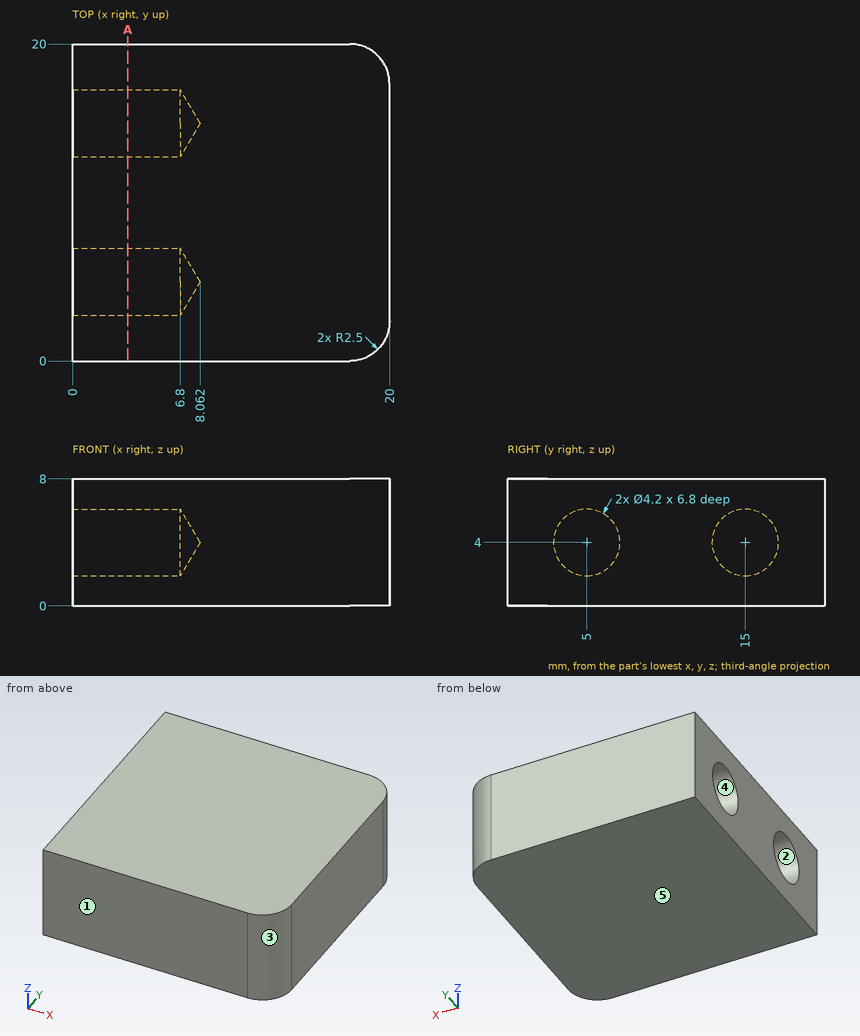
Verification items for this drawing (mm, ordinates from the low corner). A direction names the side the tool comes from. Coordinates: 2 decimals unless noted, no trailing zeros. Order: outer loops, then holes, each group sorted by start corner. A loop starts at its lowest first (then second) coordinate and runs counter-clockwise, first axis right, second up. Notation, with made-up numbers: (-5.75, 66.25) -> (35.25, 66.25) arc R13 cw to (35.25, 91.25) -> close; hole circle Ø6 at (-0.75, -30). An arc over 180 degrees is marked (long way). Answer as CSV lines item,"result". Start each with the question number.
1) Material ranges on L1, parallel to Y at x = 2, z = 4; L2, parallel to Z at x = 4, y = 15; L3, parallel to Z at x = 7.5, y = 14.5, recorded low to high. Write a range as [from, to].
2) Release check for a two-part mould opening along Y. For the marked faces 3, 4 and 5 record: released by +Y, released by -Y, zero draft, split by the parting line, or undercut.
3) Set-up check for the marked faces 1 and 2: record each of +Z, -Z, +X, -X, +Y, -Y from which the full face is reachable in a straight line by a thin tool's end or side.
4) Cross-section at A-A, the plane x = 3.5. Record the boundary of the cut face in (y, z).
5) Gauge pin test, flat ends, axial feed: pin 1 Ø1 at (y, z) = (18, 2) entering from -X; pin 2 Ø3.5 at (y, z) = (15, 4) entering from -X. Record the tip position at first contact, or that the pin passes through.
Conclusion:
1,L1,"y = [0, 2.9], [7.1, 12.9], [17.1, 20]"
1,L2,"z = [0, 1.9], [6.1, 8]"
1,L3,"z = [0, 3.21], [4.79, 8]"
2,face 3,"released by -Y"
2,face 4,"undercut"
2,face 5,"zero draft"
3,face 1,"+Z, -Z, +X, -X, -Y"
3,face 2,"-X"
4,outline,"(0, 0) -> (20, 0) -> (20, 8) -> (0, 8) -> close; hole circle Ø4.2 at (5, 4); hole circle Ø4.2 at (15, 4)"
5,pin 1,"stops at x = 0"
5,pin 2,"stops at x = 7.01"
